from build123d import *

# Parameters (mm, degrees)
CROQUIS1_R              = 4.7625
SALIENTE_EXTRUIR1_DEPTH = 113
CROQUIS2_R              = 2.38125
CORTAR_EXTRUIR1_DEPTH   = 10


with BuildPart() as part:
    # Croquis1 → Saliente-Extruir1 (new body)
    with BuildSketch(Plane(origin=(0, 0, 0), x_dir=(1, 0, 0), z_dir=(0, 1, 0))):
        with Locations(Location((0, 0, 0), (0, 0, 270))):
            Circle(CROQUIS1_R)
    extrude(amount=SALIENTE_EXTRUIR1_DEPTH)

    # Croquis2 → Cortar-Extruir1 (cut)
    with BuildSketch(Plane(origin=(0, 113, 0), x_dir=(1, 0, 0), z_dir=(0, 1, 0))):
        with Locations(Location((0, 0, 0), (0, 0, 270))):
            Circle(CROQUIS2_R)
    cortar_extruir1 = extrude(amount=-CORTAR_EXTRUIR1_DEPTH, mode=Mode.SUBTRACT)

    # Simetría1: Cortar-Extruir1 across plane
    add(cortar_extruir1.mirror(Plane.ZX.offset(56.5)), mode=Mode.SUBTRACT)


solid = part.part
Check sheet for the modelled part. Datum: model origin and axes. Units: mm. A direction names the side the tool comes from. Give positions to 0.01 mm unless a question says otherwise; leave off trailing zeros. Write each loop counter-clockwise with the first axis right and the second up, starting at its lowest first coordinate (ties: lowest second). Pieces come first, ordered by that corner, then holes. Notation, with made-up numbers: (64.5, 84.5) -> (110.5, 84.5) arc R4 cw to (110.5, 88.5) -> close; hole circle Ø7 at (62.5, -4.75). An arc over 180 degrees is marked (long way). Use one line per item in the form item = value. Start each with the question number.
1. Section check A-A (x = 0). Record the cut outline in (y, z), and give its area (3 significant figures).
2. Thickness scan on line 1 along X through (y, z) = (108.5, 0); line 2 along Z through (x, y) = (-0.25, 51.5); line 3 along X through (y, z) = (8, 0.5). Record the ranges inside material, lowest first. Write a range as from..to.
3. Mould release check, pull along Y, two halves, no side actions. Record for faces 1 (the flat face through (-2, 113, 2)), 2 (the flat face through (-2, 0, 2)), 3 (the cylindrical face through (-1.45, 4.93, -1.89)): pulls with the +Y half, pulls with the -Y half, needs draft (parallel to the pull), parting line crosses it, or undercut.
4. Access from +Z, -Z, +X, -X, +Y, -Y to the whole of each face (thin tool, end or side, straight path). Record for faces 4 (the flat face through (0, 10, 0)), 5 (the cylindrical face through (-2.9, 55.71, -3.78)), 6 (the flat face through (0, 103, 0)).
5. Go/stop test with flat-tipped pins: P1, Ø1.5, axis at x = 1.5, z = 0.5, coming from the +Y side; P2, Ø2, axis at x = 1.5, y = 77.5, coming from the +Z side; P3, Ø2, axis at x = 3, y = 80.5, coming from the +Z side. Record where each tip stops, or that it passes through.
6. Section check B-B (z = 0). Record the cut outline in (x, y), and give its area (3 significant figures).
7. Section check C-C (y = 94.5). Record the cut outline in (x, z) (1 decimal).
Conclusion:
q1.outline = (0, -4.76) -> (113, -4.76) -> (113, -2.38) -> (103, -2.38) -> (103, 2.38) -> (113, 2.38) -> (113, 4.76) -> (0, 4.76) -> (0, 2.38) -> (10, 2.38) -> (10, -2.38) -> (0, -2.38) -> close
q1.area = 981 mm²
q2.line_1 = -4.76..-2.38, 2.38..4.76
q2.line_2 = -4.76..4.76
q2.line_3 = -4.74..-2.33, 2.33..4.74
q3.face_1 = pulls with the +Y half
q3.face_2 = pulls with the -Y half
q3.face_3 = needs draft
q4.face_4 = -Y
q4.face_5 = +Y, -Y
q4.face_6 = +Y
q5.P1 = 103
q5.P2 = 4.74
q5.P3 = 4.32
q6.outline = (-4.76, 0) -> (-2.38, 0) -> (-2.38, 10) -> (2.38, 10) -> (2.38, 0) -> (4.76, 0) -> (4.76, 113) -> (2.38, 113) -> (2.38, 103) -> (-2.38, 103) -> (-2.38, 113) -> (-4.76, 113) -> close
q6.area = 981 mm²
q7.outline = circle Ø9.5 at (0, 0)
